```python
from build123d import *

# Parameters (mm, degrees)
BOSS_EXTRUDE1_DEPTH = 180
SKETCH2_R           = 2.5
CUT_EXTRUDE1_DEPTH  = 180
FILLET1_R           = 1


with BuildPart() as part:
    # Sketch1 → Boss-Extrude1 (new body)
    with BuildSketch(Plane.XY):
        Polygon((0, 0), (30, 0), (30, 100), (28, 100), (28, 2), (0, 2), align=None)
    extrude(amount=BOSS_EXTRUDE1_DEPTH)

    # Sketch2 → Cut-Extrude1 (cut)
    with BuildSketch(Plane(origin=(30, 0, 0), x_dir=(0, 0, -1), z_dir=(1, 0, 0))):
        with Locations((-122, 50)):
            Circle(SKETCH2_R)
        with Locations((-122, 18)):
            Circle(SKETCH2_R)
        with Locations((-158, 18)):
            Circle(SKETCH2_R)
        with Locations((-158, 50)):
            Circle(SKETCH2_R)
        Polygon((0, 0), (0, 100), (-40.402622584, 100), align=None)
    extrude(amount=-CUT_EXTRUDE1_DEPTH, mode=Mode.SUBTRACT)

    # Fillet1
    fillet1_edges = [part.edges().sort_by_distance(p)[0] for p in [
        (30, 0, 90),
    ]]
    fillet(fillet1_edges, radius=FILLET1_R)


solid = part.part
```
Check sheet for the modelled part. Datum: model origin and axes. Units: mm. Round coordinates to 2 decimals unless told otherwise and drop trailing zeros. Order: outer loops, then holes, each group sorted by start corner. A loop starts at its lowest first (then second) coordinate and runs counter-clockwise, first axis right, second up. Notation, with made-up numbers: (-38.75, -5.5) -> (-14.75, -5.5) arc R10 cw to (-14.75, 9.5) -> close; hole circle Ø10 at (68.5, 22.5). An arc over 180 degrees is marked (long way). One line per item, written item: value. Start each with the question number.
Q1. Cross-section at C-C (z = 54). Record the boundary of the cut face in (x, y).
Q2. Gauge pin test, flat ends, axial feed: pin 1 Ø3 at (y, z) = (86.5, 108) entering from -X; pin 2 Ø3 at (y, z) = (18, 158) entering from -X; pin 3 Ø4 at (x, z) = (13, 152) entering from +Y. Record the tip position at first contact, or that the pin passes through.
Q3. Cross-section at D-D (x = 12). Record the boundary of the cut face in (y, z).
Q4. Mould release check, pull along Y, two halves, no side actions. Record for faces 1 (the face through (28, 52, 109)), 2 (the face through (14, 2, 89)), 3 (the face through (29.014, 18.751, 119.615)): pulls with the +Y half, pulls with the -Y half, needs draft (parallel to the pull), parting line crosses it, or undercut.
Q5. Cross-section at A-A (z = 158). Record the boundary of the cut face in (x, y).
Q6. Cross-section at B-B (y = 50). Record the boundary of the cut face in (x, z), and give its area (3 significant figures).
Q7. Thickness scan on line 1 (Y direction, x = 29.1, z = 158); line 2 (Y direction, x = 29.4, z = 122); line 3 (Y direction, x = 10, z = 10.5). Record the ranges inside material, lowest first.
Completed:
1. outline: (0, 0) -> (29, 0) arc R1 ccw to (30, 1) -> (30, 100) -> (28, 100) -> (28, 2) -> (0, 2) -> close
2. pin 1: stops at x = 28
2. pin 2: passes through
2. pin 3: stops at y = 2
3. outline: (0, 0) -> (2, 0.81) -> (2, 180) -> (0, 180) -> close
4. face 1: needs draft
4. face 2: pulls with the +Y half
4. face 3: undercut
5. outline: (0, 0) -> (29, 0) arc R1 ccw to (30, 1) -> (30, 15.5) -> (28, 15.5) -> (28, 2) -> (0, 2) -> close; (28, 20.5) -> (30, 20.5) -> (30, 47.5) -> (28, 47.5) -> close; (28, 52.5) -> (30, 52.5) -> (30, 100) -> (28, 100) -> close
6. outline: (28, 20.2) -> (30, 20.2) -> (30, 119.5) -> (28, 119.5) -> close; (28, 124.5) -> (30, 124.5) -> (30, 155.5) -> (28, 155.5) -> close; (28, 160.5) -> (30, 160.5) -> (30, 180) -> (28, 180) -> close
6. area: 300 mm²
7. line 1: y = 0.01 to 15.5, 20.5 to 47.5, 52.5 to 100
7. line 2: y = 0.08 to 15.5, 20.5 to 47.5, 52.5 to 100
7. line 3: y = 0 to 2
